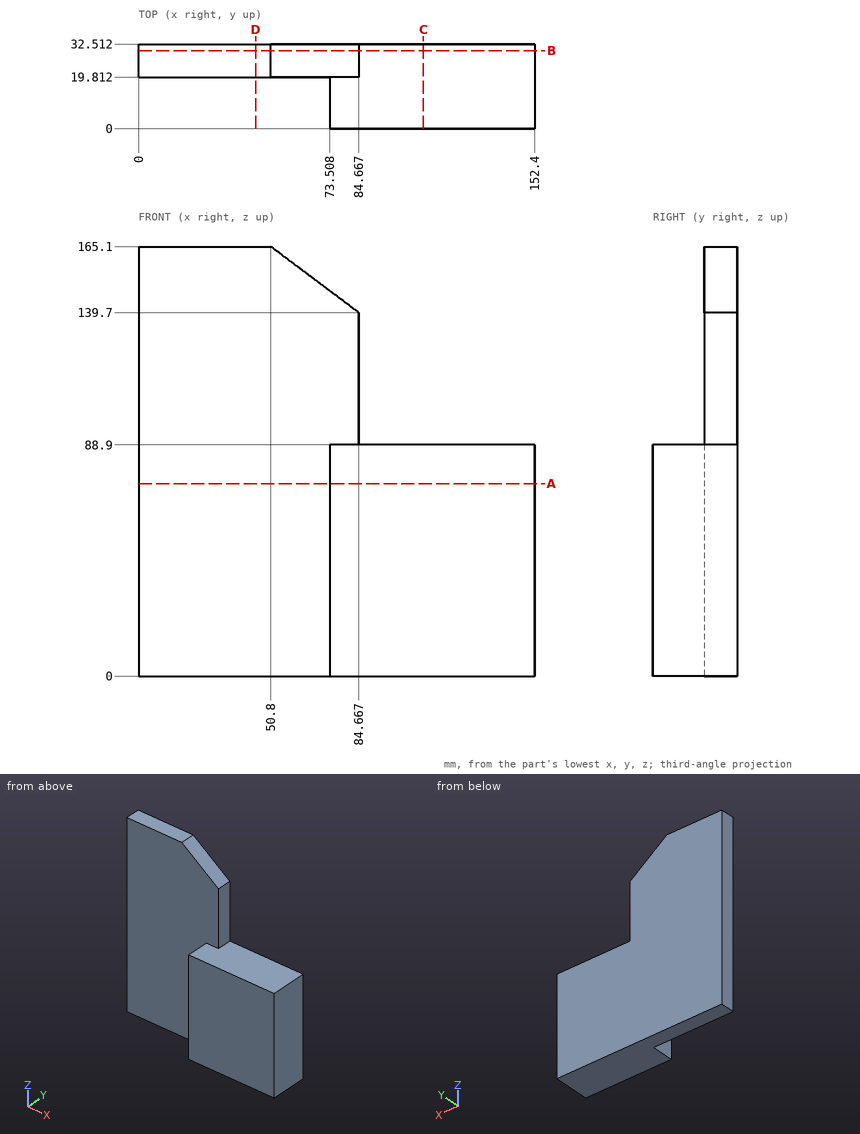
The drawing under review shows one solid part. Ordinate dimensions are in mm from its lowest x, y, z. Round coordinates to 2 decimals unless told otherwise and drop trailing zeros. Order: outer loops, then holes, each group sorted by start corner. A loop starts at its lowest first (then second) coordinate and runs counter-clockwise, first axis right, second up. Notation, with made-up numbers: (72.5, 79) - (121.5, 79) arc R14 ccw to (121.5, 83) - close; hole circle Ø10 at (13.25, 79). An arc over 180 degrees is marked (long way). Return JSON: item names as keys, results as strings.
Q1. For pin 1 Ø2 at (x, y) = (82, 8.5) entering from +Z; pin 2 Ø4 at (y, z) = (25.5, 112) entering from +X; pin 3 Ø10 at (y, z) = (5, 65.5) entering from -X, all flat-tipped, find the tip position at first contact; note any pin that passes through.
Computed values:
{"pin 1": "stops at z = 88.9", "pin 2": "stops at x = 84.67", "pin 3": "stops at x = 73.51"}
Q2. Consider section B-B on y = 30. Write out the cut boundary in (x, z).
Computed values:
{"outline": "(0, 0) - (152.4, 0) - (152.4, 88.9) - (84.67, 88.9) - (84.67, 139.7) - (50.8, 165.1) - (0, 165.1) - close"}
Q3. Wall thickness on L1, parallel to Y at x = 40, z = 126; L2, parallel to Z at x = 91, y = 23; L3, parallel to X at y = 16.5, z = 48: over which ranges is each line inside the solid? List them lowest first. Write a range as [from, to].
Computed values:
{"L1": "y = [19.81, 32.51]", "L2": "z = [0, 88.9]", "L3": "x = [73.51, 152.4]"}
Q4. Consider section D-D on x = 45. Write out the cut boundary in (y, z), plus the area to 3 significant figures.
Computed values:
{"outline": "(19.81, 0) - (32.51, 0) - (32.51, 165.1) - (19.81, 165.1) - close", "area": "2,100 mm2"}
Q5. Consider section A-A on z = 74. Write out the cut boundary in (x, y), plus the area to 3 significant figures.
Computed values:
{"outline": "(0, 19.81) - (73.51, 19.81) - (73.51, 0) - (152.4, 0) - (152.4, 32.51) - (0, 32.51) - close", "area": "3,500 mm2"}
Q6. Consider section C-C on x = 109.5. Write out the cut boundary in (y, z), plus the area to 3 significant figures.
Computed values:
{"outline": "(0, 0) - (32.51, 0) - (32.51, 88.9) - (0, 88.9) - close", "area": "2,890 mm2"}
